Work out the finished part from the listing and answer in its coordinate system (mm). Round coordinates to 2 decimals unless told otherwise and drop trailing zeros. Order: outer loops, then holes, each group sorted by start corner. A loop starts at its lowest first (then second) coordinate and runs counter-clockwise, first axis right, second up. Notation, with made-up numbers: M -24,40.5 L 30,40.5 A34 ccw 30,78.5 Z; hole C 72,32 d10. An arc over 180 degrees is marked long. Return JSON: item names as keys, results as strings.
from build123d import *

# Parameters (mm, degrees)
SKETCH_W     = 50
SKETCH_H     = 50
PAD_DEPTH    = 5
SKETCH001_R  = 5
POCKET_DEPTH = 3


with BuildPart() as part:
    # Sketch → Pad (new body)
    with BuildSketch(Plane.XY):
        Rectangle(SKETCH_W, SKETCH_H)
    extrude(amount=PAD_DEPTH)

    # Sketch001 (on Face6 of Pad) → Pocket (cut)
    with BuildSketch(Plane.XY.offset(5)):
        with Locations((-14.29406, 13.309855)):
            Circle(SKETCH001_R)
    pocket = extrude(amount=-POCKET_DEPTH, mode=Mode.SUBTRACT)

    # Mirrored: Pocket across Sketch001 V_Axis
    add(pocket.mirror(Plane(origin=(0, 0, 5), x_dir=(0, 0, 1), z_dir=(1, 0, 0))), mode=Mode.SUBTRACT)


solid = part.part
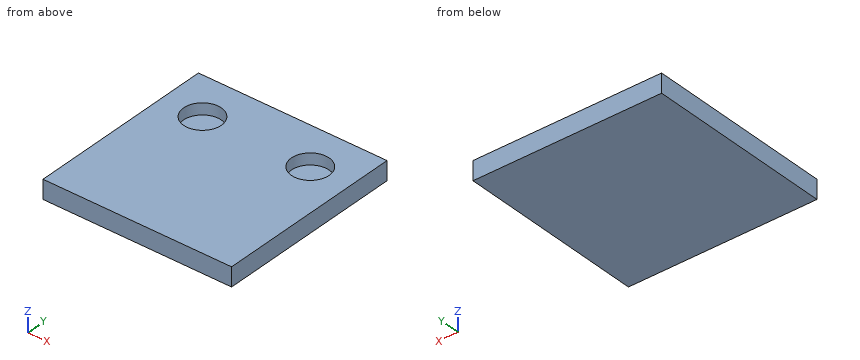
Item 1: Find section C-C (x = 14.5). Determine the outline of the cut face in (y, z).
Output:
{"outline": "M -25,0 L 25,0 L 25,5 L 18.31,5 L 18.31,2 L 8.31,2 L 8.31,5 L -25,5 Z"}
Item 2: Consider line 1 along X through (y, z) = (14, 4.1); line 2 along Y through (x, z) = (14.5, 3.8); line 3 along Y through (x, z) = (-18.5, 2.8). Determine where each line is inside the solid, lowest interval first. Write a range as [from, to].
Output:
{"line 1": "x = [-25, -19.25], [-9.34, 9.34], [19.25, 25]", "line 2": "y = [-25, 8.31], [18.31, 25]", "line 3": "y = [-25, 10.61], [16.01, 25]"}
Item 3: This flat-tipped pin is pushed along its axis until it touches: pin 1 (5 mm diameter, centred on x = -14.5, y = 14, fed in from +Z). Where does it stop, or does it pass through?
Output:
{"pin 1": "stops at z = 2"}
Item 4: Find section B-B (z = 2.65). Determine the outline of the cut face in (x, y), plus the area to 3 significant figures.
Output:
{"outline": "M -25,-25 L 25,-25 L 25,25 L -25,25 Z; hole C -14.29,13.31 d10; hole C 14.29,13.31 d10", "area": "2,340 mm^2"}
Item 5: Find section A-A (x = -10). Determine the outline of the cut face in (y, z), plus the area to 3 significant figures.
Output:
{"outline": "M -25,0 L 25,0 L 25,5 L 15.87,5 L 15.87,2 L 10.75,2 L 10.75,5 L -25,5 Z", "area": "235 mm^2"}
